Input: part model. Units: mm. Frame: model coordinates. Face numbers are marked on the shaded views. Coordinates: 2 decimals unless noted, no trailing zeros. Write each loop counter-clockwise with the first axis right and the second up, starting at its lowest first coordinate (ties: lowest second). Pieces come first, ordered by that corner, then holes. Notation, with made-up numbers: M 67,-18 L 93,-18 A26 ccw 93,16 Z; hole C 0,-20.75 d11. An arc over 180 degrees is marked long. Use one line per item in the form item = value.
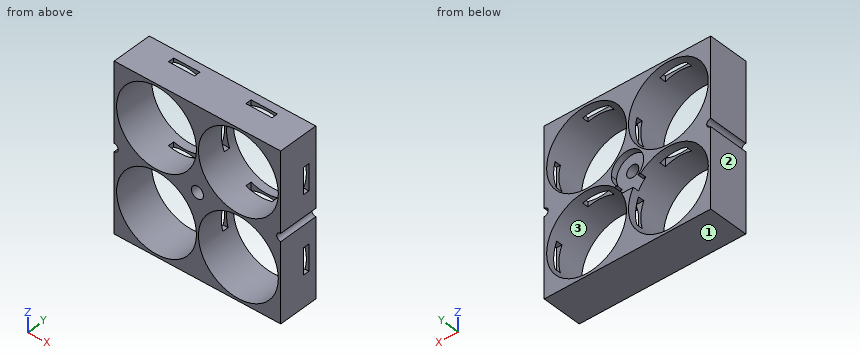
from build123d import *

# Parameters (mm, degrees)
CROQUIS1_R              = 9.9
SALIENTE_EXTRUIR1_DEPTH = 10
CROQUIS3_W              = 6.5
CROQUIS3_H              = 1.5
CORTAR_EXTRUIR1_DEPTH   = 26
MATRIZC1_COUNT          = 2
MATRIZC1_ANGLE          = 90
CORTAR_EXTRUIR3_DEPTH   = 1.5
CROQUIS6_R              = 1.5
CORTAR_EXTRUIR4_DEPTH   = 48.5


with BuildPart() as part:
    # Croquis1 → Saliente-Extruir1 (new body)
    with BuildSketch(Plane(origin=(0, 0, 0), x_dir=(1, 0, 0), z_dir=(0, 1, 0))):
        with BuildLine():
            Line((20.65, 20.65), (-20.65, 20.65))
            Line((-20.65, 20.65), (-20.65, 1))
            ThreePointArc((-20.65, 1), (-19.942893219, 0.707106781), (-19.65, 0))
            ThreePointArc((-19.65, 0), (-19.942893219, -0.707106781), (-20.65, -1))
            Line((-20.65, -1), (-20.65, -20.65))
            Line((-20.65, -20.65), (20.65, -20.65))
            Line((20.65, -20.65), (20.65, -1))
            ThreePointArc((20.65, -1), (19.65, 0), (20.65, 1))
            Line((20.65, 1), (20.65, 20.65))
        make_face()
        with Locations((-10.15, -10.15)):
            Circle(CROQUIS1_R, mode=Mode.SUBTRACT)
        with Locations((10.15, -10.15)):
            Circle(CROQUIS1_R, mode=Mode.SUBTRACT)
        with Locations((-10.15, 10.15)):
            Circle(CROQUIS1_R, mode=Mode.SUBTRACT)
        with Locations((10.15, 10.15)):
            Circle(CROQUIS1_R, mode=Mode.SUBTRACT)
    extrude(amount=SALIENTE_EXTRUIR1_DEPTH)

    # Croquis3 → Cortar-Extruir1 (cut)
    with BuildSketch(Plane.XY.offset(20.65)):
        with Locations((-9.6, 7.25)):
            Rectangle(CROQUIS3_W, CROQUIS3_H)
        with Locations((9.6, 7.25)):
            Rectangle(CROQUIS3_W, CROQUIS3_H)
    cortar_extruir1 = extrude(amount=-CORTAR_EXTRUIR1_DEPTH, mode=Mode.SUBTRACT)

    # MatrizC1: Cortar-Extruir1 ×2 about axis
    matrizc1_axis = Axis((0, 25.469690993, 0), (0, 1, 0))
    for i in range(1, MATRIZC1_COUNT):
        add(cortar_extruir1.rotate(matrizc1_axis, i * MATRIZC1_ANGLE / (MATRIZC1_COUNT - 1)), mode=Mode.SUBTRACT)

    # Croquis5 → Cortar-Extruir3 (cut)
    with BuildSketch(Plane(origin=(0, 10, 0), x_dir=(1, 0, 0), z_dir=(0, 1, 0))):
        with BuildLine():
            ThreePointArc((4, 0), (3.623813236, 1.693510446), (2.566011184, 3.068482785))
            Line((2.566011184, 3.068482785), (-2.566011184, 3.068482785))
            ThreePointArc((-2.566011184, 3.068482785), (-1.693510446, -3.623813236), (4, 0))
        make_face()
        with BuildLine():
            Line((-2.566011184, 3.068482785), (2.566011184, 3.068482785))
            ThreePointArc((2.566011184, 3.068482785), (0, 4), (-2.566011184, 3.068482785))
        make_face()
        with BuildLine():
            ThreePointArc((3.231754996, 3.068482785), (2.238589759, 4.198564207), (1.428132105, 5.466089196))
            Line((1.428132105, 5.466089196), (-1.428132105, 5.466089196))
            ThreePointArc((-1.428132105, 5.466089196), (-2.238589759, 4.198564207), (-3.231754996, 3.068482785))
            Line((-3.231754996, 3.068482785), (-2.566011184, 3.068482785))
            ThreePointArc((-2.566011184, 3.068482785), (0, 4), (2.566011184, 3.068482785))
            Line((2.566011184, 3.068482785), (3.231754996, 3.068482785))
        make_face()
    extrude(amount=-CORTAR_EXTRUIR3_DEPTH, mode=Mode.SUBTRACT)

    # Croquis6 → Cortar-Extruir4 (cut)
    with BuildSketch(Plane(origin=(0, 8.5, 0), x_dir=(1, 0, 0), z_dir=(0, 1, 0))):
        Circle(CROQUIS6_R)
    extrude(amount=-CORTAR_EXTRUIR4_DEPTH, mode=Mode.SUBTRACT)


solid = part.part
(1) Section query D-D on z = 15.5. Return the cut outline in (x, y), plus the area to 3 significant figures.
Computed:
outline = M -20.65,0 L -18.48,0 L -18.48,10 L -20.65,10 Z; M -1.82,0 L 1.82,0 L 1.82,10 L -1.82,10 Z; M 18.48,0 L 20.65,0 L 20.65,10 L 18.48,10 Z
area = 79.8 mm^2
(2) First-contact query: pin 1 Ø0.6 at (y, z) = (7, 0) entering from -X; pin 2 Ø5 at (x, z) = (0, 0) entering from +Y. Flat tips, straight axial feed; report the tip coordinate or a pass-through.
Computed:
pin_1 = -19.7
pin_2 = 8.5
(3) Section query C-C on z = -10.15. Return the cut outline in (x, y), plus the area to 4 significant figures.
Computed:
outline = M -20.65,0 L -20.05,0 L -20.05,10 L -20.65,10 Z; M -0.25,0 L 0.25,0 L 0.25,6.5 L -0.25,6.5 Z; M -0.25,8 L 0.25,8 L 0.25,10 L -0.25,10 Z; M 20.05,0 L 20.65,0 L 20.65,6.5 L 20.05,6.5 Z; M 20.05,8 L 20.65,8 L 20.65,10 L 20.05,10 Z
area = 15.35 mm^2
(4) Section query A-A on x = 10.15. Return the cut outline in (y, z).
Computed:
outline = M 0,-20.65 L 10,-20.65 L 10,-20.05 L 0,-20.05 Z; M 0,-0.25 L 6.5,-0.25 L 6.5,0.25 L 0,0.25 Z; M 0,20.05 L 6.5,20.05 L 6.5,20.65 L 0,20.65 Z; M 8,-0.25 L 10,-0.25 L 10,0.25 L 8,0.25 Z; M 8,20.05 L 10,20.05 L 10,20.65 L 8,20.65 Z
(5) Section query B-B on y = 1.25. Return the cut outline in (x, z).
Computed:
outline = M -20.65,-20.65 L 20.65,-20.65 L 20.65,-1 A1 cw 20.65,1 L 20.65,20.65 L -20.65,20.65 L -20.65,1 A1 cw -20.65,-1 Z; hole C -10.15,-10.15 d19.8; hole C -10.15,10.15 d19.8; hole C 0,0 d3; hole C 10.15,-10.15 d19.8; hole C 10.15,10.15 d19.8
(6) Pull-direction query (Z, two-part tool) for the marked faces 1, 2 and 3; classes: pulls with the +Z half, pulls with the -Z half, needs draft (parallel to the pull), parting line crosses it, or undercut.
Computed:
face_1 = pulls with the -Z half
face_2 = needs draft
face_3 = undercut
(7) Line query: probe 1 along X at (y, z) = (4.25, 10.15); probe 2 along X at (y, z) = (3, 0); probe 3 along Z at (x, y) = (10.5, 1.75). Output: solid intervals per line, ascending.
Computed:
probe_1 = -20.65 to -20.05, -0.25 to 0.25, 20.05 to 20.65
probe_2 = -19.65 to -1.5, 1.5 to 19.65
probe_3 = -20.65 to -20.04, -0.26 to 0.26, 20.04 to 20.65
